Can you work these out from the drawing? Everything is in mm from the part's minimum corner. A direction names the side the tool comes from. Give positions to 0.01 mm unless a question says otherwise; leave off trailing zeros. Write each loop counter-clockwise with the first axis right and the second up, starting at its lowest first coordinate (ties: lowest second). Pieces come first, ordered by that corner, then holes. Notation, with made-up numbers: (-4.5, -29.5) -> (7.5, -29.5) arc R28 ccw to (7.5, -10.5) -> close; hole circle Ø7 at (38.25, 31). An arc over 180 degrees is marked (long way). Return JSON: item names as keys, results as strings.
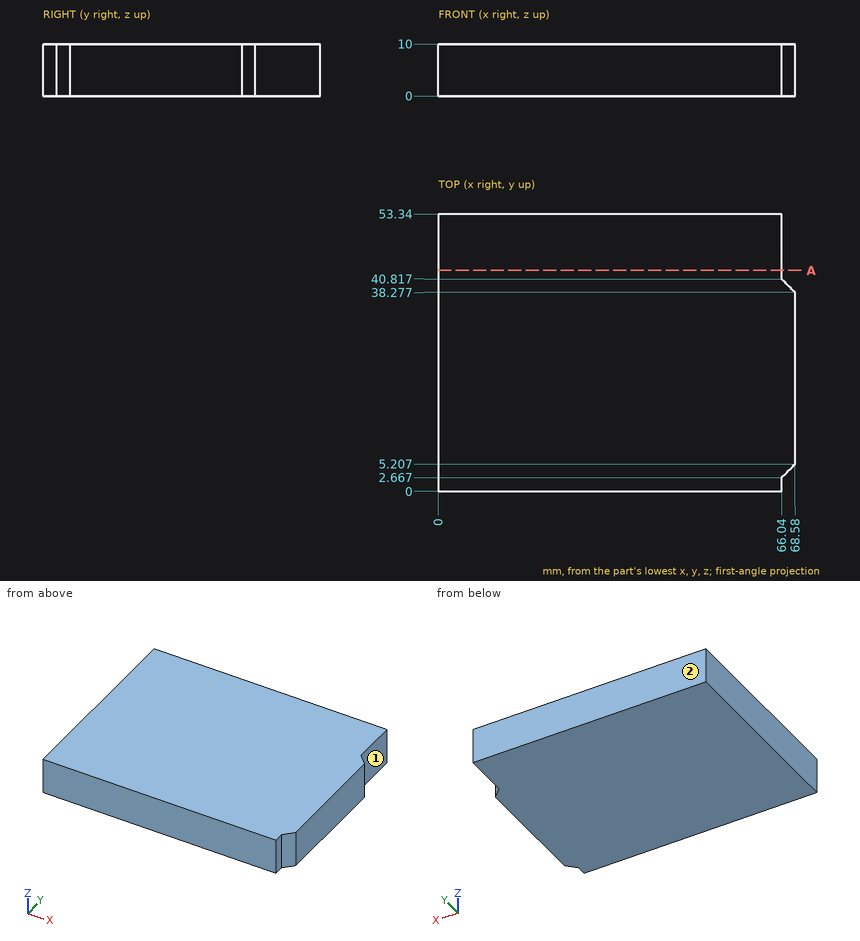
1. For pin 1 Ø0.8 at (y, z) = (1, 4.5) entering from +X, with a flat end and sliding along its axis, tell me the tip position at first contact or that it passes through.
Taken from the geometry:
{"pin 1": "stops at x = 66.04"}
2. If I drill on line 1 (X direction, y = 41.5, z = 7); line 2 (X direction, y = 40.5, z = 4), over which ranges is the centre line in solid material (lowest first)? Write a range as [from, to].
Taken from the geometry:
{"line 1": "x = [0, 66.04]", "line 2": "x = [0, 66.36]"}
3. Suppose I cut it at A-A, the plane y = 42.5. List the corners of the cut face in (x, z) for me.
Taken from the geometry:
{"outline": "(0, 0) -> (66.04, 0) -> (66.04, 10) -> (0, 10) -> close"}
4. Which directions (+Z, -Z, +X, -X, +Y, -Y) give clear straight access to the entire face, cutting with the end or side of a thin tool? Please do the marked faces 1 and 2.
Taken from the geometry:
{"face 1": "+Z, -Z, +X, +Y", "face 2": "+Z, -Z, +X, -X, +Y"}
